Can you work these out from the model? Positions are in its coordinate system, mm. Coordinates: 2 decimals unless noted, no trailing zeros. Order: outer loops, then holes, each group sorted by start corner. A loop starts at its lowest first (then second) coordinate and runs counter-clockwise, first axis right, second up. Notation, with made-up numbers: (74, 24) -> (133, 24) arc R20 cw to (133, 59) -> close; hole circle Ø5 at (11, 85.25). An arc over 180 degrees is marked (long way). Write item = value, one per line. Start each with the question number.
from build123d import *

# Parameters (mm, degrees)
SKETCH1_W           = 50
SKETCH1_H           = 33.876964868
BOSS_EXTRUDE1_DEPTH = 3
SKETCH2_R           = 1
SKETCH2_W           = 24
SKETCH2_H           = 13
CUT_EXTRUDE1_DEPTH  = 4


with BuildPart() as part:
    # Sketch1 → Boss-Extrude1 (new body)
    with BuildSketch(Plane(origin=(0, 0, 0), x_dir=(0, 0, -1), z_dir=(1, 0, 0))):
        with Locations((16.038383019, -39.775181141)):
            Rectangle(SKETCH1_W, SKETCH1_H)
    extrude(amount=BOSS_EXTRUDE1_DEPTH)

    # Sketch2 → Cut-Extrude1 (cut, through all)
    with BuildSketch(Plane.ZY):
        with Locations((-35.020353647, -45.551677475)):
            Circle(SKETCH2_R)
        with Locations((-7.220353647, -45.551677475)):
            Circle(SKETCH2_R)
        with Locations((-35.020353647, -32.293971569)):
            Circle(SKETCH2_R)
        with Locations((-7.220353647, -32.293971569)):
            Circle(SKETCH2_R)
        with Locations((-21.120353647, -45.551677475)):
            Rectangle(SKETCH2_W, SKETCH2_H)
        with Locations((-21.120353647, -32.293971569)):
            Rectangle(SKETCH2_W, SKETCH2_H)
    extrude(amount=-CUT_EXTRUDE1_DEPTH, mode=Mode.SUBTRACT)


solid = part.part
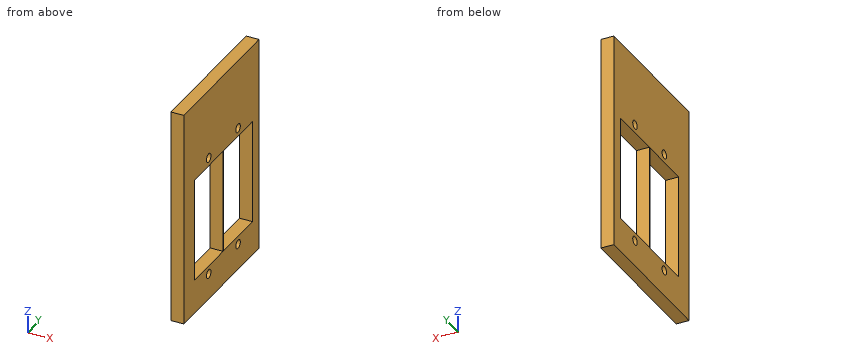
(1) Imagine slicing it at A-A (z = -24.5). Write out the boundary of the cut face in (x, y).
(2) Imagine slicing it at D-D (z = -7). Write out the boundary of the cut face in (x, y), plus the area to 3 significant figures.
(3) Imagine slicing it at C-C (x = 2.55). Write out the boundary of the cut face in (y, z).
(4) For P1, Ø1.6, axis at y = -32.29, z = -35.02, coming from the -X side, with a flat end and sliding along its axis, tell me the tip position at first contact or that it passes through.
(5) If I drill on L1, parallel to Y at x = 0.2, z = -31.5; L2, parallel to Z at x = 2.4, y = -44; L3, parallel to Z at x = 0.8, y = -33, over which ranges is the centre line in solid material (lowest first)? Write a range as from..to.
(6) Imagine slicing it at B-B (y = -34). Write out the boundary of the cut face in (x, z), plus the area to 3 significant figures.
Result set:
q1.outline = (0, -56.71) -> (3, -56.71) -> (3, -52.05) -> (0, -52.05) -> close; (0, -39.05) -> (3, -39.05) -> (3, -38.79) -> (0, -38.79) -> close; (0, -25.79) -> (3, -25.79) -> (3, -22.84) -> (0, -22.84) -> close
q2.outline = (0, -56.71) -> (3, -56.71) -> (3, -46.53) -> (0, -46.53) -> close; (0, -44.58) -> (3, -44.58) -> (3, -33.27) -> (0, -33.27) -> close; (0, -31.32) -> (3, -31.32) -> (3, -22.84) -> (0, -22.84) -> close
q2.area = 89.9 mm2
q3.outline = (-56.71, -41.04) -> (-22.84, -41.04) -> (-22.84, 8.96) -> (-56.71, 8.96) -> close; hole (-52.05, -33.12) -> (-39.05, -33.12) -> (-39.05, -9.12) -> (-52.05, -9.12) -> close; hole circle Ø2 at (-45.55, -35.02); hole circle Ø2 at (-45.55, -7.22); hole (-38.79, -33.12) -> (-25.79, -33.12) -> (-25.79, -9.12) -> (-38.79, -9.12) -> close; hole circle Ø2 at (-32.29, -35.02); hole circle Ø2 at (-32.29, -7.22)
q4.P1 = through
q5.L1 = -56.71..-52.05, -39.05..-38.79, -25.79..-22.84
q5.L2 = -41.04..-33.12, -9.12..8.96
q5.L3 = -41.04..-35.73, -34.31..-33.12, -9.12..-7.93, -6.51..8.96
q6.outline = (0, -41.04) -> (3, -41.04) -> (3, -33.12) -> (0, -33.12) -> close; (0, -9.12) -> (3, -9.12) -> (3, 8.96) -> (0, 8.96) -> close
q6.area = 78.0 mm2
